Here's how the part is built. I have some questions about the finished solid (model axes, mm). A direction names the side the tool comes from. Round coordinates to 2 decimals unless told otherwise and drop trailing zeros. Order: outer loops, then holes, each group sorted by start corner. A loop starts at its lowest first (then second) coordinate and runs counter-clockwise, first axis right, second up. Notation, with made-up numbers: (50, 82.5) -> (56, 82.5) arc R17 cw to (56, 100.5) -> close; hole circle Ø10 at (-10, -2). An arc over 180 degrees is marked (long way). One line per item, written item: value.
Autodesk Inventor part; units mm, degrees
ref_plane "YZ Plane" through (0, 0, 0) normal (1, 0, 0) x (0, 1, 0)
ref_plane "XZ Plane" through (0, 0, 0) normal (0, 1, 0) x (-1, 0, 0)
ref_plane "XY Plane" through (0, 0, 0) normal (0, 0, 1) x (1, 0, 0)
sketch "Sketch1" plane through (0, 0, 0) normal (1, 0, 0) x (0, 1, 0)
  line L0 (1.056781, -0.379193) -> (0.980627, -0.195884)
  line L1 (1.056781, -0.379193) -> (1.12494, -0.418544)
  line L2 (1.12494, -0.418544) -> (0.92494, -0.764955)
  line L3 (0.92494, -0.764955) -> (0.856781, -0.725603)
  line L4 (0.659954, -0.751306) -> (0.856781, -0.725603)
  arc A0 (0.320673, -0.94719) -> (0.659954, -0.751306) centre (0, 0) ccw
  line L5 (0.2, -1.104796) -> (0.320673, -0.94719)
  line L6 (0.2, -1.104796) -> (0.2, -1.183499)
  line L7 (0.2, -1.183499) -> (-0.2, -1.183499)
  line L8 (-0.2, -1.183499) -> (-0.2, -1.104796)
  line L9 (-0.320673, -0.94719) -> (-0.2, -1.104796)
  arc A1 (-0.659954, -0.751306) -> (-0.320673, -0.94719) centre (0, 0) ccw
  line L10 (-0.856781, -0.725603) -> (-0.659954, -0.751306)
  line L11 (-0.856781, -0.725603) -> (-0.92494, -0.764955)
  line L12 (-0.92494, -0.764955) -> (-1.12494, -0.418544)
  line L13 (-1.12494, -0.418544) -> (-1.056781, -0.379193)
  line L14 (-0.980627, -0.195884) -> (-1.056781, -0.379193)
  arc A2 (-0.980627, 0.195884) -> (-0.980627, -0.195884) centre (0, 0) ccw
  line L15 (-1.056781, 0.379193) -> (-0.980627, 0.195884)
  line L16 (-1.056781, 0.379193) -> (-1.12494, 0.418544)
  line L17 (-1.12494, 0.418544) -> (-0.92494, 0.764955)
  line L18 (-0.92494, 0.764955) -> (-0.856781, 0.725603)
  line L19 (-0.659954, 0.751306) -> (-0.856781, 0.725603)
  arc A3 (-0.320673, 0.94719) -> (-0.659954, 0.751306) centre (0, 0) ccw
  line L20 (-0.2, 1.104796) -> (-0.320673, 0.94719)
  line L21 (-0.2, 1.104796) -> (-0.2, 1.183499)
  line L22 (-0.2, 1.183499) -> (0.2, 1.183499)
  line L23 (0.2, 1.183499) -> (0.2, 1.104796)
  line L24 (0.320673, 0.94719) -> (0.2, 1.104796)
  arc A4 (0.659954, 0.751306) -> (0.320673, 0.94719) centre (0, 0) ccw
  line L25 (0.856781, 0.725603) -> (0.659954, 0.751306)
  line L26 (0.856781, 0.725603) -> (0.92494, 0.764955)
  line L27 (0.92494, 0.764955) -> (1.12494, 0.418544)
  line L28 (1.12494, 0.418544) -> (1.056781, 0.379193)
  line L29 (0.980627, 0.195884) -> (1.056781, 0.379193)
  arc A5 (0.980627, -0.195884) -> (0.980627, 0.195884) centre (0, 0) ccw
  circle A6 centre (0, 0) radius 1.469987
  point P0 (0, 0)
extrude "Extrusion1" add sketch "Sketch1" against normal blind 3 contours L1 L2 L3 L4 A0 L5 L6 L7 L8 L9 A1 L10 L11 L12 L13 L14 A2 L15 L16 L17 L18 L19 A3 L20 L21 L22 L23 L24 A4 L25 L26 L27 L28 L29 A5 L0
sketch "Sketch1 outline for Extrusion2" plane through (0, 0, 0) normal (1, 0, 0) x (0, 1, 0)
  circle A0 centre (0, 0) radius 1.469987
extrude "Extrusion2" add sketch "Sketch1 outline for Extrusion2" along normal blind 3 draft -5
sketch "Sketch2" plane through (3, 0, 0) normal (1, 0, 0) x (0, 0, -1)
  circle A0 centre (0, 0) radius 0.7
  dimension "d6" = 1.4
extrude "Extrusion3" add sketch "Sketch2" along normal blind 2.5
sketch "Sketch3" plane through (5.5, 0, 0) normal (1, 0, 0) x (0, 0, -1)
  circle A0 centre (0, 0) radius 1
  dimension "d7" = 2
extrude "Extrusion4" add sketch "Sketch3" along normal blind 4
sketch "Sketch4" plane through (9.5, 0, 0) normal (1, 0, 0) x (0, 0, -1)
  circle A0 centre (0, 0) radius 0.8
  line L0 (0, -0.8) -> (-0.69282, -0.4)
  line L1 (-0.69282, -0.4) -> (-0.69282, 0.4)
  line L2 (-0.69282, 0.4) -> (0, 0.8)
  line L3 (0, 0.8) -> (0.69282, 0.4)
  line L4 (0.69282, 0.4) -> (0.69282, -0.4)
  line L5 (0.69282, -0.4) -> (0, -0.8)
  dimension "d10" = 1.6
extrude "Extrusion5" cut sketch "Sketch4" against normal blind 3 contours L4 L5 L0 L1 L2 L3
fillet "Fillet1" radius 0.2 4 edges at (5.5, 0, 1) (3, -1.2075, 0) (3, 0, 0.7) (5.5, 0, 0.7)
sketch "Sketch5" plane through (-3, 0, 0) normal (-1, 0, 0) x (0, 0, 1)
  circle A0 centre (0, 0) radius 0.37
  dimension "d14" = 0.74
extrude "Extrusion6" add sketch "Sketch5" along normal blind 0.5
thread "Thread1"
properties part number "lagnut_screw" material "Steel"
Q1. I want a section at B-B on x = 5. Write out the boundary of the cut face in (y, z), then the cut area to 3 significant figures.
Answers:
outline: circle Ø1.4 at (0, 0)
area: 1.54 mm2
Q2. I want a section at C-C on x = 1.75. Write out the boundary of the cut face in (y, z).
Answers:
outline: circle Ø2.63 at (0, 0)
Q3. For P1, Ø0.6, axis at x = 8.5, y = 0, coming from the +Z side; P2, Ø1.5, axis at x = 3.5, z = 0.5, coming from the -Y side; P3, Ø0.9, axis at x = 8, y = 0, coming from the -Z side, each with a flat end and sliding along its axis, tell me the tip position at first contact or that it passes through.
Answers:
P1: z = 1
P2: y = -1.21
P3: z = -1
Q4. If we mould it in two halves opening along Z, with no side actions, what happens to faces 1 (the face through (-3, 0.5, -0.2)), 2 (the face through (6.5, 0, 0)), 3 (the face through (8, 1, 0))? For each: pulls with the +Z half, pulls with the -Z half, needs draft (parallel to the pull), parting line crosses it, or undercut.
Answers:
face 1: needs draft
face 2: undercut
face 3: parting line crosses it
Q5. I need wall thicknesses on line 1 along Z through (x, y) = (7, 0.05); line 2 along X through (y, z) = (1.05, -0.1); line 3 along X through (y, z) = (0.1, 0.65). Which ranges of each line are inside material? Lowest first, please.
Answers:
line 1: -1 to -0.69, 0.69 to 1
line 2: 0 to 3
line 3: -3 to 6.5
Q6. Which directions (+Z, -Z, +X, -X, +Y, -Y) give clear straight access to the entire face, cutting with the end or side of a thin tool? Please do faces 4 (the face through (1.39, -1.07, 0.82)), 5 (the face through (4.2, 0, 0.7)).
Answers:
face 4: +X
face 5: none
